The listing builds one solid part. Answer for the finished solid, in the listing's coordinates (mm). A direction names the side the tool comes from. Give positions to 0.01 mm unless a question says otherwise; leave off trailing zeros. Write each loop counter-clockwise with the first axis right and the second up, starting at its lowest first coordinate (ties: lowest second). Pieces come first, ordered by that corner, then holes. Notation, with made-up numbers: (42, -35) - (91, -35) arc R36 ccw to (91, 4) - close; hole circle Ø4 at (-7.5, 46). An arc over 180 degrees is marked (long way). Write each question's results on one line, items separated by ' | '. Start each with the question number.
Q1. Find the intervals of material crossed by probe 1 along X at (y, z) = (1383.5, 5); probe 2 along Y at (x, z) = (288, 3.5); probe 3 along Y at (x, z) = (80, 1.5), in increasing order.
Q2. Section B-B (y = 993) is taken. Determine the outline of the cut face in (x, z).
Q3. Section A-A (z = 4) is taken. State how many separate pieces and enclosed holes the cut face has, plus the area to 3 significant figures.
Q4. Section D-D (x = 338.5) is taken. Determine the outline of the cut face in (y, z).
Q5. For faces 1 (the face through (-361, 759, 9.5)), 2 (the face through (361, 759, 9.5)), 3 (the face through (-5, 1051, 0)), determine the directions among +Z, -Z, +X, -X, +Y, -Y from which every point of the face is accessible in a straight line to the end or side of a thin tool.
Q6. Flat-ended cylindrical pins translate along their axes: pin 1 Ø3 at (y, z) = (8, 5) entering from -X; pin 2 Ø6 at (x, z) = (285.5, 6.5) entering from -Y; pin 3 Ø2 at (x, z) = (-112.5, 7.5) entering from +Y; pin 4 Ø5 at (y, z) = (2058.5, 7.5) entering from +X. Find the tip coordinate at first contact, or state that the pin passes through.
Q7. Section C-C (x = -94.5) is taken. Determine the outline of the cut face in (y, z), plus the area to 3 significant figures.
```python
from build123d import *

# Parameters (mm, degrees)
BOSS_EXTRUDE1_DEPTH = 10.16
CUT_LOFT1_DEPTH     = 9.5


# Read off the part's stored shape, not the designer's step: Cut-Loft1
with BuildPart() as part:
    # Sketch1 → Boss-Extrude1 (new body)
    # profile 1 of 2: a face of its own
    with BuildSketch(Plane.XY):
        Polygon((205.715298803, 2072.64), (123.444, 2072.64), (123.444, 2052.32), (41.135649402, 2052.32), (41.135649402, 2072.64), (-41.135649402, 2072.64), (-41.135649402, 2052.32), (-123.444, 2052.32), (-123.444, 2072.64), (-205.715298803, 2072.64), (-205.715298803, 2052.32), (-215.881789204, 2052.32), (-215.881789204, 1963.42), (-205.715298803, 1963.42), (-205.715298803, 1874.52), (-215.881789204, 1874.52), (-215.881789204, 1785.62), (-205.715298803, 1785.62), (-205.715298803, 1696.72), (-215.875298803, 1696.72), (-215.875298803, 1607.82), (-205.715298803, 1607.82), (-205.715298803, 1518.92), (205.715298803, 1518.92), (205.715298803, 1607.82), (215.875298803, 1607.82), (215.875298803, 1696.72), (205.715298803, 1696.72), (205.715298803, 1785.62), (215.881789204, 1785.62), (215.881789204, 1874.52), (205.715298803, 1874.52), (205.715298803, 1963.42), (215.881789204, 1963.42), (215.881789204, 2052.32), (205.715298803, 2052.32), align=None)
    # profile 2 of 2: a face of its own
    with BuildSketch(Plane.XY):
        Polygon((215.881789204, 1518.92), (205.715298803, 1518.92), (-205.715298803, 1518.92), (-215.881789204, 1518.92), (-215.881789204, 1476.636861244), (-402.149872815, 1476.636861244), (-358.672996954, 20.32), (-303.52, 20.32), (-303.52, 0), (-252, 0), (-252, 20.32), (-55.8292, 20.32), (-55.8292, 0), (55.8292, 0), (55.8292, 20.32), (252, 20.32), (252, 0), (303.52, 0), (303.52, 20.32), (358.672996954, 20.32), (402.149872815, 1476.636861244), (215.881789204, 1476.636861244), align=None)
        Polygon((-308.266124544, 132.94397688), (-301.755453134, 226.680843836), (-291.63777305, 225.978101227), (-298.14844446, 132.241234271), align=None, mode=Mode.SUBTRACT)
        Polygon((-289.435698895, 404.053512688), (-279.318018811, 403.350770078), (-285.830533081, 309.587370692), (-295.948213166, 310.290113301), align=None, mode=Mode.SUBTRACT)
        Polygon((-283.630301787, 487.636249721), (-277.115944656, 581.426181539), (-266.998264572, 580.72343893), (-273.512621703, 486.933507112), align=None, mode=Mode.SUBTRACT)
        Polygon((-264.796190418, 758.798850391), (-254.678510334, 758.096107781), (-261.194710324, 664.279643533), (-271.312390408, 664.982386142), align=None, mode=Mode.SUBTRACT)
        Polygon((-252.476436179, 936.171519242), (-242.358756095, 935.468776633), (-248.876798945, 841.625779953), (-258.99447903, 842.328522563), align=None, mode=Mode.SUBTRACT)
        Polygon((301.755453134, 226.680843836), (308.266124544, 132.94397688), (298.14844446, 132.241234271), (291.63777305, 225.978101227), align=None, mode=Mode.SUBTRACT)
        Polygon((279.318018811, 403.350770078), (289.435698895, 404.053512688), (295.948213166, 310.290113301), (285.830533081, 309.587370692), align=None, mode=Mode.SUBTRACT)
        Polygon((277.115944656, 581.426181539), (283.630301787, 487.636249721), (273.512621703, 486.933507112), (266.998264572, 580.72343893), align=None, mode=Mode.SUBTRACT)
        Polygon((254.678510334, 758.096107781), (264.796190418, 758.798850391), (271.312390408, 664.982386142), (261.194710324, 664.279643533), align=None, mode=Mode.SUBTRACT)
        Polygon((242.358756095, 935.468776633), (252.476436179, 936.171519242), (258.99447903, 842.328522563), (248.876798945, 841.625779953), align=None, mode=Mode.SUBTRACT)
        Polygon((-240.15668194, 1113.544188093), (-230.039001856, 1112.841445484), (-236.558887567, 1018.971916374), (-246.676567651, 1019.674658983), align=None, mode=Mode.SUBTRACT)
        Polygon((-227.836927701, 1290.916856945), (-217.719247617, 1290.214114336), (-224.240976188, 1196.318052795), (-234.358656272, 1197.020795404), align=None, mode=Mode.SUBTRACT)
        Polygon((-215.881789204, 1463.040000035), (-214.479068593, 1463.040000035), (-205.715298803, 1463.040000035), (-211.92306481, 1373.664189215), (-222.040744894, 1374.366931824), align=None, mode=Mode.SUBTRACT)
        Polygon((230.039001856, 1112.841445484), (240.15668194, 1113.544188093), (246.676567651, 1019.674658983), (236.558887567, 1018.971916374), align=None, mode=Mode.SUBTRACT)
        Polygon((217.719247617, 1290.214114336), (227.836927701, 1290.916856945), (234.358656272, 1197.020795404), (224.240976188, 1196.318052795), align=None, mode=Mode.SUBTRACT)
        Polygon((205.715298803, 1463.040000035), (215.881789204, 1463.040000035), (222.040744894, 1374.366931824), (211.92306481, 1373.664189215), align=None, mode=Mode.SUBTRACT)
    extrude(amount=BOSS_EXTRUDE1_DEPTH)

    # Cut-Loft1 outline → Cut-Loft1 (cut)
    with BuildSketch(Plane.XY):
        Polygon((402.149872815, 1476.636861244), (364.049872815, 1476.636861244), (320.627659668, 20.32), (358.672996954, 20.32), align=None)
    cut_loft1 = extrude(amount=CUT_LOFT1_DEPTH, mode=Mode.SUBTRACT)

    # Mirror1: Cut-Loft1 across plane
    add(cut_loft1.mirror(Plane(origin=(0, 0, 0), x_dir=(0, 0, 1), z_dir=(1, 0, 0))), mode=Mode.SUBTRACT)


solid = part.part
```
Answers below:
1) probe 1: x = -361.27 to -221.41, -211.24 to 211.24, 221.41 to 361.27 | probe 2: y = 0 to 309.74, 403.95 to 1476.64 | probe 3: y = 20.32 to 2052.32
2) outline: (-387.71, 9.5) - (-349.63, 9.5) - (-349.63, 0) - (349.63, 0) - (349.63, 9.5) - (387.71, 9.5) - (387.71, 10.16) - (-387.71, 10.16) - close
3) separate pieces: 1 | enclosed holes: 16 | area: 1,230,000 mm2
4) outline: (20.32, 9.5) - (619.73, 9.5) - (619.73, 0) - (1476.64, 0) - (1476.64, 10.16) - (20.32, 10.16) - close
5) face 1: -Z, -X, -Y | face 2: -Z, +X, -Y | face 3: -Z, +X, -X, +Y, -Y
6) pin 1: stops at x = -303.52 | pin 2: stops at y = 0 | pin 3: stops at y = 2052.32 | pin 4: stops at x = 205.72
7) outline: (20.32, 0) - (2052.32, 0) - (2052.32, 10.16) - (20.32, 10.16) - close | area: 20,600 mm2
